Geometry check sheet. Reference: drawing and pictorial views, mm from the part's lowest x, y, z. A direction names the side the tool comes from. Round coordinates to 2 decimals unless told otherwise and drop trailing zeros. Write each loop counter-clockwise with the first axis right and the second up, starting at its lowest first coordinate (ties: lowest second). Pieces come first, ordered by that corner, then holes. Notation, with made-up numbers: (-36, -25.5) - (-9, -25.5) arc R32 ccw to (-9, 2.5) - close; hole circle Ø6 at (83, 36.25). An arc over 180 degrees is marked (long way). Return JSON: item names as keys, results as strings.
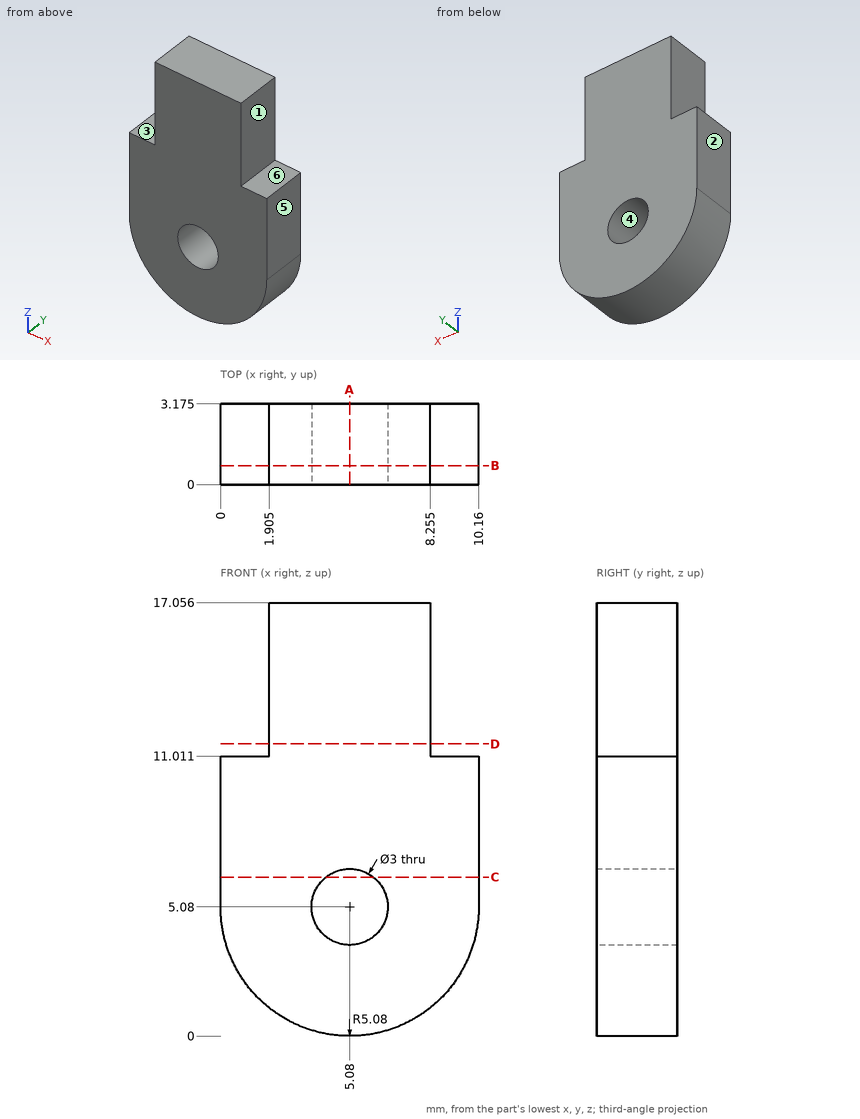
(1) Gauge pin test, flat ends, axial feed: pin 1 (1 mm diameter, centred on x = 9.5, y = 1, fed in from +Z); pin 2 (1.6 mm diameter, centred on y = 2.5, z = 13.5, fed in from -X) (3 decimals). Record the tip position at first contact, or that the pin passes through.
Response values:
{"pin 1": "stops at z = 11.01", "pin 2": "stops at x = 1.905"}
(2) Release check for a two-part mould opening along X. For the marked faces 4, 5 and 6 record: pulls with the +X half, pulls with the -X half, needs draft (parallel to the pull), parting line crosses it, or undercut.
Response values:
{"face 4": "undercut", "face 5": "pulls with the +X half", "face 6": "needs draft"}
(3) Access from +Z, -Z, +X, -X, +Y, -Y to the whole of each face (thin tool, end or side, straight path). Record for the marked faces 1, 2 and 3.
Response values:
{"face 1": "+Z, +X, +Y, -Y", "face 2": "+Z, -Z, -X, +Y, -Y", "face 3": "+Z, -X, +Y, -Y"}
(4) Section check A-A, the plane x = 5.08. Enter the section's corners in (y, z) (3 decimals), plus the area to 3 significant figures.
Response values:
{"outline": "(0, 0) - (3.175, 0) - (3.175, 3.58) - (0, 3.58) - close; (0, 6.58) - (3.175, 6.58) - (3.175, 17.056) - (0, 17.056) - close", "area": "44.6 mm^2"}
(5) Material ranges on line 1 along X through (y, z) = (0.85, 5.08); line 2 along X through (y, z) = (1, 12.25) (3 decimals); line 3 along Z through (x, y) = (5.5, 2.4), recorded low to high. Write a range as [from, to].
Response values:
{"line 1": "x = [0, 3.58], [6.58, 10.16]", "line 2": "x = [1.905, 8.255]", "line 3": "z = [0.02, 3.64], [6.52, 17.06]"}
(6) Section check C-C, the plane z = 6.25. Enter the section's corners in (x, y) (1 decimal).
Response values:
{"outline": "(0, 0) - (4.1, 0) - (4.1, 3.2) - (0, 3.2) - close; (6, 0) - (10.2, 0) - (10.2, 3.2) - (6, 3.2) - close"}
(7) Section check B-B, the plane y = 0.75. Enter the section's corners in (x, z) (3 decimals), plus the area to 3 significant figures.
Response values:
{"outline": "(0, 5.08) arc R5.08 ccw to (10.16, 5.08) - (10.16, 11.011) - (8.255, 11.011) - (8.255, 17.056) - (1.905, 17.056) - (1.905, 11.011) - (0, 11.011) - close; hole circle Ø3 at (5.08, 5.08)", "area": "132 mm^2"}
(8) Section check D-D, the plane z = 11.5. Enter the section's corners in (x, y) (3 decimals).
Response values:
{"outline": "(1.905, 0) - (8.255, 0) - (8.255, 3.175) - (1.905, 3.175) - close"}
